The listing builds one solid part. Answer for the finished solid, in the listing's coordinates (mm). A direction names the side the tool comes from. Round coordinates to 2 decimals unless told otherwise and drop trailing zeros. Order: outer loops, then holes, each group sorted by start corner. A loop starts at its lowest first (then second) coordinate and runs counter-clockwise, first axis right, second up. Notation, with made-up numbers: (76.5, 73.5) - (88.5, 73.5) arc R21 ccw to (88.5, 97.5) - close; hole circle Ø3 at (-16.75, 50). An arc over 180 degrees is marked (long way). Use CSV: the item, a comma, the result in double quotes. Start each with the question number.
Item 1: Find section B-B, the plane x = 133.35. Give the vertices of the cut face in (y, z), plus the area to 3 significant figures.
Item 2: Flat-ended cylindrical pins translate along their axes: P1, Ø8, axis at y = 15, z = -26, coming from the -X side; P2, Ø1.5, axis at y = 7.5, z = -22, coming from the +X side; P3, Ø5, axis at y = 12, z = -29.5, coming from the -X side; P4, Ø4, axis at x = 31.75, y = 19.05, coming from the +Z side. Find the tip coordinate at first contact, or state that the pin passes through.
Item 3: Find section A-A, the plane y = 12.7. Count the separate pieces of the cut face and the enclosed holes in it, plus the area to 3 significant figures.
Item 4: Determine the mould class of faces 3 (the cylindrical face through (4.777, 0.285, -35.543)), 4 (the cylindrical face through (30.712, 17.054, -38.17)), 5 (the cylindrical face through (133.838, 10.504, -38.17)), 6 (the flat face through (11.45, 12.54, -28.48)) for opening direction X: +X half, -X half, draft (parallel to the pull), parting line (faces both ways), or undercut.
Item 5: Find section C-C, the plane z = -12.7. Give the vertices of the cut face in (x, y), plus the area to 3 significant figures.
Item 6: Find section D-D, the plane x = 31.75. Give the vertices of the cut face in (y, z), plus the area to 3 significant figures.
Item 7: Straight lines are drawn through the part: line 1 along Y through (x, z) = (31.75, -35.75); line 2 along X through (y, z) = (22.75, -37); line 3 along X through (y, z) = (18.75, 0). For each, find the intervals that lie inside material, in ascending order. Write a range as [from, to].
Item 8: For faces 1 (the flat face through (87, 13, -33.1)), 2 (the flat face through (71, 25.4, -36)), determine the directions among +Z, -Z, +X, -X, +Y, -Y from which every point of the face is accessible in a straight line to the end or side of a thin tool.
```python
from build123d import *

# Parameters (mm, degrees)
SKETCH1_R           = 2.25
BOSS_EXTRUDE1_DEPTH = 25.4
FILLET2_R           = 5
CUT_EXTRUDE2_REACH  = 170.202
SKETCH3_R           = 2.25
FILLET4_R           = 12.7
FILLET5_R           = 1


with BuildPart() as part:
    # Sketch1 → Boss-Extrude1 (new body)
    # profile 1 of 2: a face of its own
    with BuildSketch(Plane(origin=(0, 0, 0), x_dir=(1, 0, 0), z_dir=(0, 1, 0))):
        Polygon((158.75, 33.1), (158.75, 43.1), (13.315419455, 43.1), (-5, 27.731538291), (-5, -6.35), (5, -6.35), (5, 23.068461709), (5, 33.1), (16.955121797, 33.1), align=None)
        with Locations(Location((0, 0, 0), (0, 0, 270))):
            Circle(SKETCH1_R, mode=Mode.SUBTRACT)
        with Locations(Location((0, 12.7, 0), (0, 0, 270))):
            Circle(SKETCH1_R, mode=Mode.SUBTRACT)
        with Locations(Location((0, 25.4, 0), (0, 0, 270))):
            Circle(SKETCH1_R, mode=Mode.SUBTRACT)
        with Locations(Location((139.7, 38.1, 0), (0, 0, 270))):
            Circle(SKETCH1_R, mode=Mode.SUBTRACT)
        with Locations(Location((152.4, 38.1, 0), (0, 0, 270))):
            Circle(SKETCH1_R, mode=Mode.SUBTRACT)
    # profile 2 of 2: a face of its own
    with BuildSketch(Plane(origin=(0, 0, 0), x_dir=(1, 0, 0), z_dir=(0, 1, 0))):
        Polygon((5, 23.068461709), (16.955121797, 33.1), (5, 33.1), align=None)
    extrude(amount=BOSS_EXTRUDE1_DEPTH)

    # Fillet2
    fillet2_edges = [part.edges().sort_by_distance(p)[0] for p in [
        (-5, 12.7, 6.35),
        (5, 12.7, 6.35),
        (158.75, 12.7, -43.1),
        (158.75, 12.7, -33.1),
    ]]
    fillet(fillet2_edges, radius=FILLET2_R - 0.0001)  # a hair under: the kernel refuses the full size

    # Sketch3 → Cut-Extrude2 (cut, up to next)
    with BuildSketch(Plane(origin=(0, 0, -43.1), x_dir=(-1, 0, 0), z_dir=(0, 0, -1)), mode=Mode.PRIVATE) as cut_extrude2_sk1:
        with Locations((-31.75, 6.35)):
            Circle(SKETCH3_R)
    cut_extrude2_tool1 = extrude(cut_extrude2_sk1.sketch, amount=-CUT_EXTRUDE2_REACH, mode=Mode.PRIVATE) & part.part
    # Sketch3 → Cut-Extrude2 (cut, up to next)
    with BuildSketch(Plane(origin=(0, 0, -43.1), x_dir=(-1, 0, 0), z_dir=(0, 0, -1)), mode=Mode.PRIVATE) as cut_extrude2_sk2:
        with Locations((-31.75, 19.05)):
            Circle(SKETCH3_R)
    cut_extrude2_tool2 = extrude(cut_extrude2_sk2.sketch, amount=-CUT_EXTRUDE2_REACH, mode=Mode.PRIVATE) & part.part
    # Sketch3 → Cut-Extrude2 (cut, up to next)
    with BuildSketch(Plane(origin=(0, 0, -43.1), x_dir=(-1, 0, 0), z_dir=(0, 0, -1)), mode=Mode.PRIVATE) as cut_extrude2_sk3:
        with Locations((-133.35, 12.7)):
            Circle(SKETCH3_R)
    cut_extrude2_tool3 = extrude(cut_extrude2_sk3.sketch, amount=-CUT_EXTRUDE2_REACH, mode=Mode.PRIVATE) & part.part
    add(cut_extrude2_tool1.solids().sort_by_distance((31.75, 6.35, -43.1))[0], mode=Mode.SUBTRACT)
    add(cut_extrude2_tool2.solids().sort_by_distance((31.75, 19.05, -43.1))[0], mode=Mode.SUBTRACT)
    add(cut_extrude2_tool3.solids().sort_by_distance((133.35, 12.7, -43.1))[0], mode=Mode.SUBTRACT)

    # Fillet4
    fillet4_edges = [part.edges().sort_by_distance(p)[0] for p in [
        (-5, 12.7, -27.731538291),
        (13.315419455, 12.7, -43.1),
        (16.955121797, 12.7, -33.1),
        (5, 12.7, -23.068461709),
    ]]
    fillet(fillet4_edges, radius=FILLET4_R)

    # Fillet5
    fillet5_edges = [part.edges().sort_by_distance(p)[0] for p in [
        (-5, 0, -10.229665516),
        (87.663821886, 0, -33.1),
        (157.285563195, 0, -34.564436805),
        (157.285563195, 0, -41.635563195),
        (3.535563195, 0, 4.885563195),
        (-3.535563195, 0, 4.885563195),
        (-5, 25.4, -10.229665516),
        (87.663821886, 25.4, -33.1),
        (157.285563195, 25.4, -34.564436805),
        (157.285563195, 25.4, -41.635563195),
        (3.535563195, 25.4, 4.885563195),
        (-3.535563195, 25.4, 4.885563195),
        (11.475369243, 0, -28.501941653),
        (11.475369243, 25.4, -28.501941653),
        (5, 25.4, -7.898127225),
        (5, 0, -7.898127225),
        (4.655518072, 0, -35.833479944),
        (4.655518072, 25.4, -35.833479944),
        (85.843970715, 0, -43.1),
        (-3.810108895, 0, -27.176682956),
        (13.59418561, 0, -42.334096284),
        (85.843970715, 25.4, -43.1),
        (-3.810108895, 25.4, -27.176682956),
        (13.59418561, 25.4, -42.334096284),
        (17.233887952, 0, -32.334096284),
        (17.233887952, 25.4, -32.334096284),
        (6.189891105, 0, -22.513606375),
        (6.189891105, 25.4, -22.513606375),
    ]]
    fillet(fillet5_edges, radius=FILLET5_R)


solid = part.part
```
Worked out:
1,outline,"(0, -42.1) arc R1 ccw to (1, -43.1) - (10.45, -43.1) - (10.45, -33.1) - (1, -33.1) arc R1 ccw to (0, -34.1) - close; (14.95, -43.1) - (24.4, -43.1) arc R1 ccw to (25.4, -42.1) - (25.4, -34.1) arc R1 ccw to (24.4, -33.1) - (14.95, -33.1) - close"
1,area,"208 mm²"
2,P1,"stops at x = -5"
2,P2,"stops at x = 6.3"
2,P3,"stops at x = -3.89"
2,P4,"passes through"
3,separate pieces,"2"
3,enclosed holes,"5"
3,area,"1,810 mm²"
4,face 3,"-X half"
4,face 4,"undercut"
4,face 5,"undercut"
4,face 6,"+X half"
5,outline,"(-5, 1) arc R1 ccw to (-4, 0) - (-2.25, 0) - (-2.25, 25.4) - (-4, 25.4) arc R1 ccw to (-5, 24.4) - close; (2.25, 0) - (4, 0) arc R1 ccw to (5, 1) - (5, 24.4) arc R1 ccw to (4, 25.4) - (2.25, 25.4) - close"
5,area,"139 mm²"
6,outline,"(0, -42.1) arc R1 ccw to (1, -43.1) - (4.1, -43.1) - (4.1, -33.1) - (1, -33.1) arc R1 ccw to (0, -34.1) - close; (8.6, -43.1) - (16.8, -43.1) - (16.8, -33.1) - (8.6, -33.1) - close; (21.3, -43.1) - (24.4, -43.1) arc R1 ccw to (25.4, -42.1) - (25.4, -34.1) arc R1 ccw to (24.4, -33.1) - (21.3, -33.1) - close"
6,area,"163 mm²"
7,line 1,"y = [0, 4.1], [8.6, 16.8], [21.3, 25.4]"
7,line 2,"x = [6.05, 137.74], [141.66, 150.44], [154.36, 158.63]"
7,line 3,"x = [-5, -2.25], [2.25, 5]"
8,face 1,"+Z, +X, +Y, -Y"
8,face 2,"+Z, -Z, +X, -X, +Y"
